```python
from build123d import *

# Parameters (mm, degrees)
F0_R     = 85.725
F1_DEPTH = 101.6
F2_R     = 82.55
F3_DEPTH = 96.52
F4_R     = 5.08
F5_R     = 3.175
F6_DEPTH = 254


with BuildPart() as f1:
    # F0 (on Front) → F1 (new body)
    with BuildSketch(Plane.XZ):
        Circle(F0_R)
    extrude(amount=-F1_DEPTH)

    # F2 (on face) → F3 (cut)
    with BuildSketch(Plane(origin=(0, 101.6, 0), x_dir=(-1, 0, 0), z_dir=(0, 1, 0))):
        Circle(F2_R)
    extrude(amount=-F3_DEPTH, mode=Mode.SUBTRACT)

    # F4
    f4_edges = [f1.edges().sort_by_distance(p)[0] for p in [
        (-85.725, 0, 0),
    ]]
    fillet(f4_edges, radius=F4_R)

    # F5 (on Top) → F6 (cut, symmetric)
    with BuildSketch(Plane.XY):
        with Locations((0, 50.8)):
            Circle(F5_R)
    extrude(amount=F6_DEPTH, both=True, mode=Mode.SUBTRACT)


solid = f1.part
```
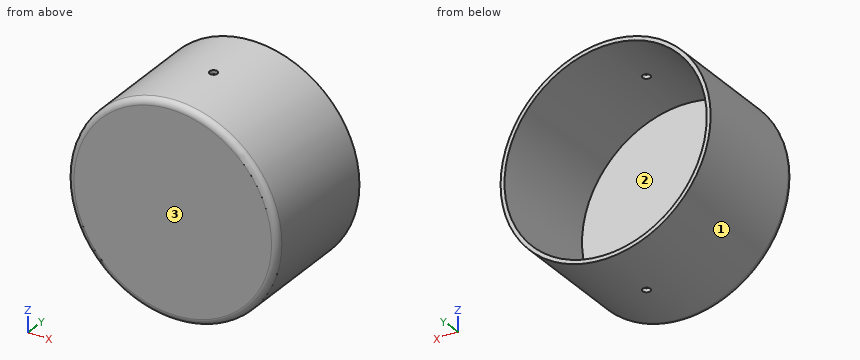
Part model, mm, in its own coordinate system. Face numbers are marked on the shaded views. Round coordinates to 2 decimals unless told otherwise and drop trailing zeros. Loops run counter-clockwise (first coordinate to the right, second up) from the corner with the lowest first, then second, coordinate; pieces in that order, holes last. Notation, with made-up numbers: (53, 63) -> (84, 63) arc R24 cw to (84, 90) -> close; hole circle Ø7 at (48, -26.5). An arc over 180 degrees is marked (long way). Use a Markdown table: item, result.
1) Cut at C-C, the plane z = 0. List the corners of the cut face in (x, y) (3 decimals), and give its area (3 significant figures).
The answers:
| item | result |
|---|---|
| outline | (-85.725, 5.08) arc R5.08 ccw to (-80.645, 0) -> (80.645, 0) arc R5.08 ccw to (85.725, 5.08) -> (85.725, 101.6) -> (82.55, 101.6) -> (82.55, 5.08) -> (-82.55, 5.08) -> (-82.55, 101.6) -> (-85.725, 101.6) -> close |
| area | 1,470 mm2 |
2) Cut at A-A, the plane x = 0. List the corners of the cut face in (y, z) (3 decimals).
The answers:
| item | result |
|---|---|
| outline | (0, -80.645) arc R5.08 ccw to (5.08, -85.725) -> (47.625, -85.725) -> (47.625, -82.55) -> (5.08, -82.55) -> (5.08, 82.55) -> (47.625, 82.55) -> (47.625, 85.725) -> (5.08, 85.725) arc R5.08 ccw to (0, 80.645) -> close; (53.975, -85.725) -> (101.6, -85.725) -> (101.6, -82.55) -> (53.975, -82.55) -> close; (53.975, 82.55) -> (101.6, 82.55) -> (101.6, 85.725) -> (53.975, 85.725) -> close |
3) Drop flat-ended pins along their axis: pin 1 Ø4 at (x, y) = (51.5, 49) entering from +Z; pin 2 Ø1 at (y, z) = (32.5, 57) entering from +X; pin 3 Ø12 at (y, z) = (75, -6.5) entering from -X. Give the stop position or say it passes through.
The answers:
| item | result |
|---|---|
| pin 1 | stops at z = 69.99 |
| pin 2 | stops at x = 64.47 |
| pin 3 | stops at x = -85.72 |
4) Pull direction X, two halves, no side cores. Call the marked faces 1, 2 and 3: pulls with the +X half, pulls with the -X half, needs draft (parallel to the pull), parting line crosses it, or undercut.
The answers:
| item | result |
|---|---|
| face 1 | parting line crosses it |
| face 2 | undercut |
| face 3 | needs draft |
5) Cut at D-D, the plane y = 35.5. List the corners of the cut face in (x, z) (3 decimals), and give its area (3 significant figures).
The answers:
| item | result |
|---|---|
| outline | circle Ø171.45 at (0, 0); hole circle Ø165.1 at (0, 0) |
| area | 1,680 mm2 |
6) Probe line 1 (Z direction, x = 0, y = 35.5) (3 decimals); line 2 (Y direction, x = 72, z = -25.5); line 3 (Z direction, x = 30, y = 22.5). List the from-to ranges inside material, lowest first. Write a range as [from, to].
The answers:
| item | result |
|---|---|
| line 1 | z = [-85.725, -82.55], [82.55, 85.725] |
| line 2 | y = [0, 5.08] |
| line 3 | z = [-80.3, -76.91], [76.91, 80.3] |
7) Cut at B-B, the plane y = 50.8. List the corners of the cut face in (x, z) (3 decimals), and give its area (3 significant figures).
The answers:
| item | result |
|---|---|
| outline | (-3.175, -85.666) -> (-3.175, -82.489) arc R82.55 cw to (-3.175, 82.489) -> (-3.175, 85.666) arc R85.725 ccw to start; (3.175, -85.666) arc R85.725 ccw to (3.175, 85.666) -> (3.175, 82.489) arc R82.55 cw to (3.175, -82.489) -> close |
| area | 1,640 mm2 |
